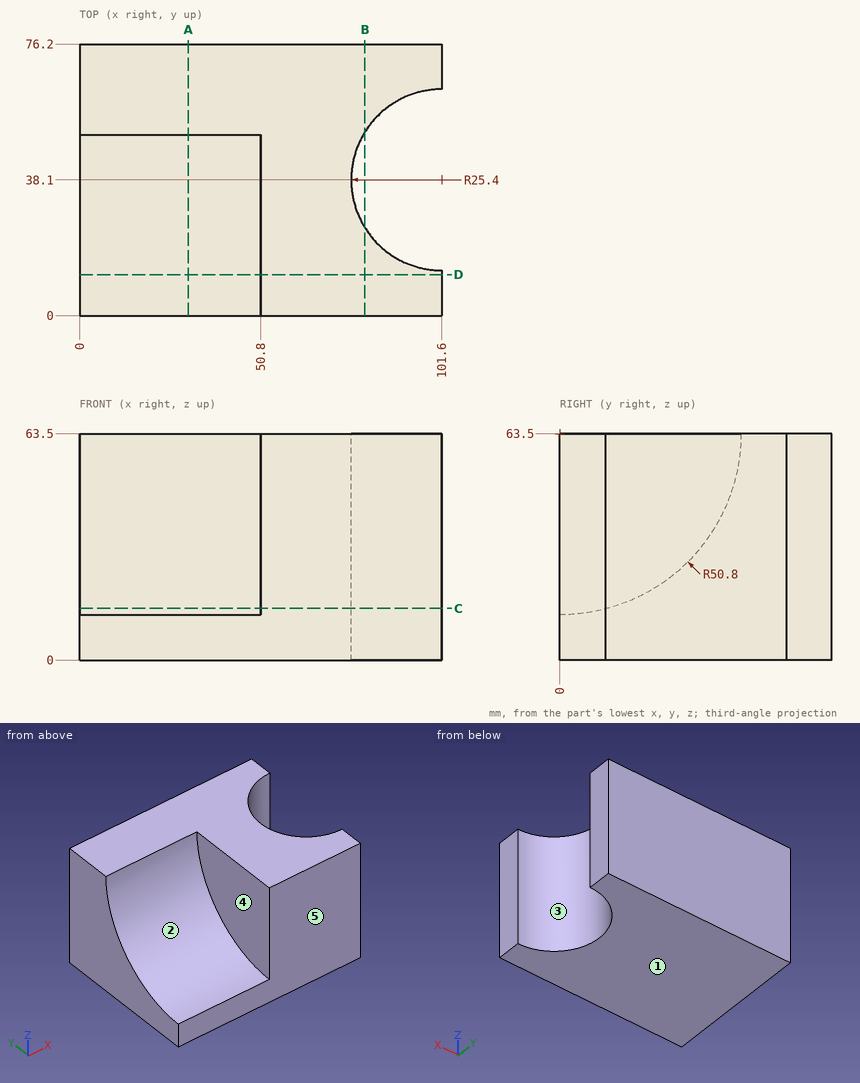
Geometry check sheet. Reference: drawing and pictorial views, mm from the part's lowest x, y, z. A direction names the side the tool comes from. Round coordinates to 2 decimals unless told otherwise and drop trailing zeros. Loops run counter-clockwise (first coordinate to the right, second up) from the corner with the lowest first, then second, coordinate; pieces in that order, holes last. Notation, with made-up numbers: (-11, 50.25) -> (-5, 50.25) arc R24 ccw to (-5, 78.25) -> close; hole circle Ø4 at (-19, -8). An arc over 180 degrees is marked (long way). Use a Markdown table: item, result.
(1) Scan lines: probe 1 along X at (y, z) = (8, 13.5); probe 2 along Y at (x, z) = (82.5, 41); probe 3 along Y at (x, z) = (78.5, 32.5). Record each from-to range of solid material in increasing order.
Calculated:
| item | result |
|---|---|
| probe 1 | 50.8 to 101.6 |
| probe 2 | 0 to 21.36, 54.84 to 76.2 |
| probe 3 | 0 to 27.54, 48.66 to 76.2 |
(2) Mould release check, pull along Y, two halves, no side actions. Record for the marked faces 3, 4 and 5: released by +Y, released by -Y, zero draft, split by the parting line, or undercut.
Calculated:
| item | result |
|---|---|
| face 3 | undercut |
| face 4 | zero draft |
| face 5 | released by -Y |
(3) Sectioned sample at D-D (y = 11.5). Enter the section's corners in (x, z), then the cut area to 3 significant figures.
Calculated:
| item | result |
|---|---|
| outline | (0, 0) -> (101.6, 0) -> (101.6, 63.5) -> (50.8, 63.5) -> (50.8, 14.02) -> (0, 14.02) -> close |
| area | 3,940 mm² |
(4) Go/stop test with flat-tipped pins: P1, Ø5, axis at y = 9.5, z = 35, coming from the -X side; P2, Ø12, axis at x = 13.5, y = 53.5, coming from the -Z side; P3, Ø1, axis at y = 28, z = 26.5, coming from the +X side. Record where each tip stops, or that it passes through.
Calculated:
| item | result |
|---|---|
| P1 | x = 50.8 |
| P2 | z = 0 |
| P3 | x = 78.52 |
(5) Sectioned sample at A-A (x = 30.5). Enter the section's corners in (y, z), then the cut area to 3 significant figures.
Calculated:
| item | result |
|---|---|
| outline | (0, 0) -> (76.2, 0) -> (76.2, 63.5) -> (50.8, 63.5) arc R50.8 cw to (0, 12.7) -> close |
| area | 2,810 mm² |
(6) Sectioned sample at B-B (x = 80). Enter the section's corners in (y, z), then the cut area to 3 significant figures.
Calculated:
| item | result |
|---|---|
| outline | (0, 0) -> (24.74, 0) -> (24.74, 63.5) -> (0, 63.5) -> close; (51.46, 0) -> (76.2, 0) -> (76.2, 63.5) -> (51.46, 63.5) -> close |
| area | 3,140 mm² |
(7) Set-up check for the marked faces 1 and 2: record each of +Z, -Z, +X, -X, +Y, -Y from which the full face is reachable in a straight line by a thin tool's end or side.
Calculated:
| item | result |
|---|---|
| face 1 | -Z, +X, -X, +Y, -Y |
| face 2 | +Z, -X, -Y |
(8) Sectioned sample at C-C (z = 14.5). Enter the section's corners in (x, y), then the cut area to 3 significant figures.
Calculated:
| item | result |
|---|---|
| outline | (0, 13.4) -> (50.8, 13.4) -> (50.8, 0) -> (101.6, 0) -> (101.6, 12.7) arc R25.4 cw to (101.6, 63.5) -> (101.6, 76.2) -> (0, 76.2) -> close |
| area | 6,050 mm² |
